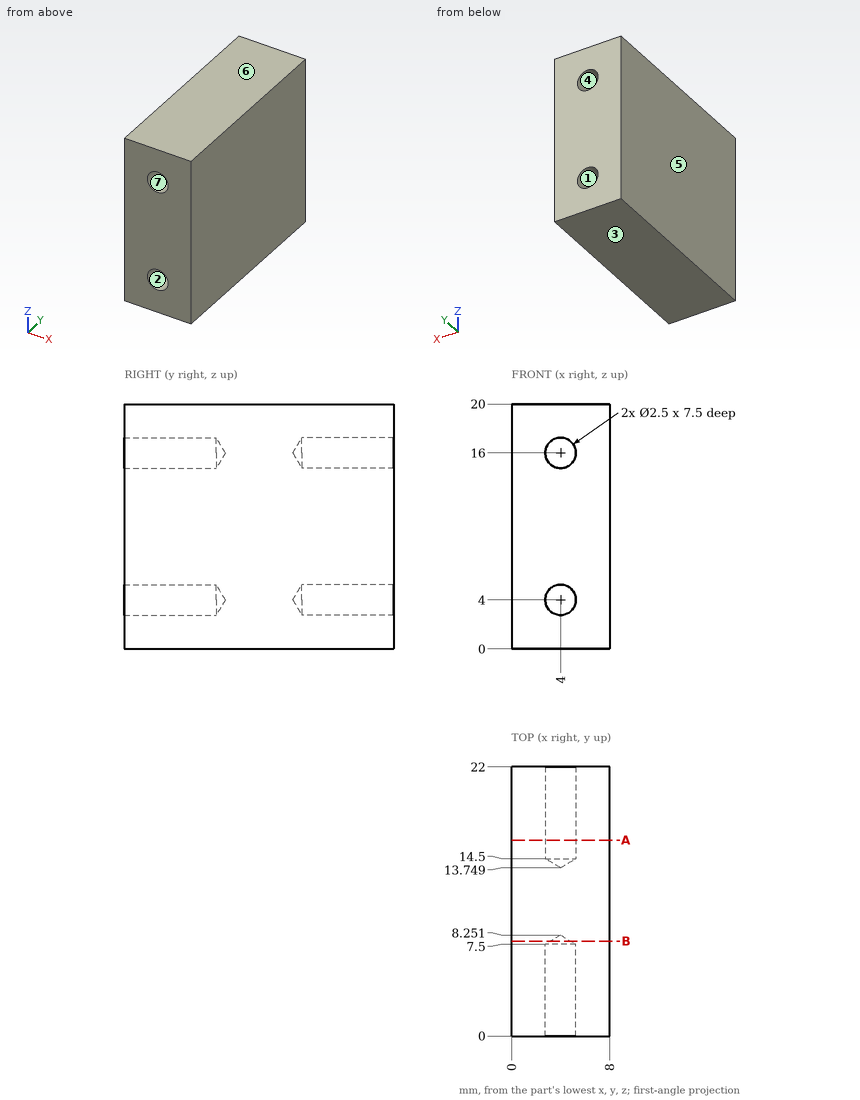
Could you check a few things on this drawing? It's one solid part, dimensions in mm from its lowest x, y, z. A direction names the side the tool comes from. Give positions to 0.01 mm unless a question says otherwise; leave off trailing zeros. Order: outer loops, then holes, each group sorted by start corner. A loop starts at its lowest first (then second) coordinate and runs counter-clockwise, first axis right, second up. Notation, with made-up numbers: (42, -1.75) - (48, -1.75) arc R16 cw to (48, 22.25) - close; hole circle Ø1 at (-37, 3.25). An arc over 180 degrees is marked (long way). One line per item, written item: value. Start each with the question number.
1. If I drill on probe 1 along Z at (x, y) = (4, 4); probe 2 along X at (y, z) = (17.25, 16); probe 3 along Z at (x, y) = (5, 16.5), over which ranges is the centre line in solid material (lowest first)?
2. Thinking about a two-plate mould opening in Z: for the marked faces 4, 5, 6 and 7, which applies, +Z half, -Z half, draft (parallel to the pull), parting line (faces both ways), or undercut?
3. Imagine slicing it at A-A on y = 16. List the corners of the cut face in (x, z) for me, plus the area to 3 significant figures.
4. For P1, Ø1.5, axis at x = 4, z = 16, coming from the -Y side, with a flat end and sliding along its axis, tell me the tip position at first contact or that it passes through.
5. For the marked faces 1, 2 and 3, which set-ups out of +Z, -Z, +X, -X, +Y, -Y let a thin tool reach every point of the face, with its end or its side?
6. Imagine slicing it at B-B on y = 7.75. List the corners of the cut face in (x, z) for me.
Values:
1. probe 1: 0 to 2.75, 5.25 to 14.75, 17.25 to 20
1. probe 2: 0 to 2.75, 5.25 to 8
1. probe 3: 0 to 3.25, 4.75 to 15.25, 16.75 to 20
2. face 4: undercut
2. face 5: draft
2. face 6: +Z half
2. face 7: undercut
3. outline: (0, 0) - (8, 0) - (8, 20) - (0, 20) - close; hole circle Ø2.5 at (4, 4); hole circle Ø2.5 at (4, 16)
3. area: 150 mm²
4. P1: y = 7.8
5. face 1: +Y
5. face 2: -Y
5. face 3: -Z, +X, -X, +Y, -Y
6. outline: (0, 0) - (8, 0) - (8, 20) - (0, 20) - close; hole circle Ø1.67 at (4, 4); hole circle Ø1.67 at (4, 16)
